```python
from build123d import *

# Parameters (mm, degrees)
SKETCH1_W                = 44.2976
SKETCH1_H                = 37.084
BOSS_EXTRUDE1_DEPTH      = 5.334
SKETCH2_W                = 6.1976
SKETCH2_H                = 5.334
CUT_EXTRUDE1_DEPTH       = 80.087198141
LPATTERN1_COUNT          = 3
LPATTERN1_PITCH          = 12.7
SKETCH3_W                = 5.334
SKETCH3_H                = 6.1976
CUT_EXTRUDE2_DEPTH       = 80.087198141
LPATTERN2_COUNT          = 2
LPATTERN2_PITCH          = 12.7
F_0_257_DIAMETER_HOLE1_D = 6.5278


with BuildPart() as part:
    # Sketch1 → Boss-Extrude1 (new body)
    with BuildSketch(Plane.XY):
        with Locations((50.0888, 13.208)):
            Rectangle(SKETCH1_W, SKETCH1_H)
    extrude(amount=-BOSS_EXTRUDE1_DEPTH)

    # Sketch2 → Cut-Extrude1 (cut, through all)
    with BuildSketch(Plane.XY):
        with Locations((62.7888, -2.667)):
            Rectangle(SKETCH2_W, SKETCH2_H)
    cut_extrude1 = extrude(amount=-CUT_EXTRUDE1_DEPTH, mode=Mode.SUBTRACT)

    # LPattern1: Cut-Extrude1 ×3
    with Locations(*[(-i * LPATTERN1_PITCH, 0, 0) for i in range(1, LPATTERN1_COUNT)]):
        add(cut_extrude1, mode=Mode.SUBTRACT)

    # Sketch3 → Cut-Extrude2 (cut, through all)
    with BuildSketch(Plane(origin=(0, 0, -5.334), x_dir=(-1, 0, 0), z_dir=(0, 0, -1))):
        with Locations((-69.5706, 9.6012)):
            Rectangle(SKETCH3_W, SKETCH3_H)
        with Locations((-30.607, 9.6012)):
            Rectangle(SKETCH3_W, SKETCH3_H)
    cut_extrude2 = extrude(amount=-CUT_EXTRUDE2_DEPTH, mode=Mode.SUBTRACT)

    # LPattern2: Cut-Extrude2 ×2
    with Locations(*[(0, i * LPATTERN2_PITCH, 0) for i in range(1, LPATTERN2_COUNT)]):
        add(cut_extrude2, mode=Mode.SUBTRACT)

    # F (0.257) Diameter Hole1 (through all)
    with Locations(Plane(origin=(0, 0, -5.334), x_dir=(-1, 0, 0), z_dir=(0, 0, -1))):
        with Locations((-59.6138, 15.875), (-40.5638, 15.875)):
            Hole(F_0_257_DIAMETER_HOLE1_D / 2)


solid = part.part
```
The model under review builds one solid part; all positions refer to its coordinate system, in mm. A direction names the side the tool comes from. Round coordinates to 2 decimals unless told otherwise and drop trailing zeros. Order: outer loops, then holes, each group sorted by start corner. A loop starts at its lowest first (then second) coordinate and runs counter-clockwise, first axis right, second up. Notation, with made-up numbers: (66.25, -14) -> (98.25, -14) arc R7 cw to (98.25, -9) -> close; hole circle Ø2 at (64.25, 8). An arc over 180 degrees is marked (long way). Use a Markdown table: item, result.
Q1. We need section D-D on y = 14.5. Write out the cut boundary in (x, z).
Values:
| item | result |
|---|---|
| outline | (27.94, -5.33) -> (37.6, -5.33) -> (37.6, 0) -> (27.94, 0) -> close; (43.52, -5.33) -> (56.65, -5.33) -> (56.65, 0) -> (43.52, 0) -> close; (62.57, -5.33) -> (72.24, -5.33) -> (72.24, 0) -> (62.57, 0) -> close |
Q2. Mouldability with a two-part tool opening along X and no side actions: class faces 4 (the flat face through (40.488, -3, -3)), 5 (the flat face through (69, -5.334, -3)), 6 (the flat face through (72.238, 16, -3)) as +X half, -X half, draft (parallel to the pull), parting line (faces both ways), or undercut.
Values:
| item | result |
|---|---|
| face 4 | undercut |
| face 5 | draft |
| face 6 | +X half |
Q3. For line 1 (Y direction, x = 67.5, z = -4.2); line 2 (X direction, y = 16.5, z = -2.6); line 3 (X direction, y = -1.5, z = -1.15), list the stretches that pass through material, from the lowest coordinate up.
Values:
| item | result |
|---|---|
| line 1 | y = -5.33 to 6.5, 12.7 to 19.2, 25.4 to 31.75 |
| line 2 | x = 27.94 to 37.36, 43.77 to 56.41, 62.82 to 72.24 |
| line 3 | x = 27.94 to 34.29, 40.49 to 46.99, 53.19 to 59.69, 65.89 to 72.24 |
Q4. Tool access review of faces 1 (the flat face through (31, 19.202, -3)), 2 (the flat face through (70, 12.7, -3)), 3 (the flat face through (63, 0, -3)): name each direction out of +Z, -Z, +X, -X, +Y, -Y from which nothing blocks a thin tool from reaching the whole face with its end or side.
Values:
| item | result |
|---|---|
| face 1 | +Z, -Z, -X |
| face 2 | +Z, -Z, +X |
| face 3 | +Z, -Z, -Y |
Q5. We need section C-C on z = -3.7. State how many separate pieces and enclosed holes the cut face has, then the cut area to 3 significant figures.
Values:
| item | result |
|---|---|
| separate pieces | 1 |
| enclosed holes | 2 |
| area | 1,340 mm^2 |
Q6. We need section B-B on x = 58.5. Write out the cut boundary in (y, z), then the cut area to 3 significant figures.
Values:
| item | result |
|---|---|
| outline | (-5.33, -5.33) -> (12.81, -5.33) -> (12.81, 0) -> (-5.33, 0) -> close; (18.94, -5.33) -> (31.75, -5.33) -> (31.75, 0) -> (18.94, 0) -> close |
| area | 165 mm^2 |
Q7. We need section A-A on y = -0.5. Write out the cut boundary in (x, z).
Values:
| item | result |
|---|---|
| outline | (27.94, -5.33) -> (34.29, -5.33) -> (34.29, 0) -> (27.94, 0) -> close; (40.49, -5.33) -> (46.99, -5.33) -> (46.99, 0) -> (40.49, 0) -> close; (53.19, -5.33) -> (59.69, -5.33) -> (59.69, 0) -> (53.19, 0) -> close; (65.89, -5.33) -> (72.24, -5.33) -> (72.24, 0) -> (65.89, 0) -> close |
Q8. Clearance check with flat-ended pins moving along their axes: P1, Ø2.5, axis at x = 36, z = -3, coming from the -Y side; P2, Ø2.5, axis at y = 10, z = -3, coming from the -X side. State where each tip first meets the part, or that it passes through.
Values:
| item | result |
|---|---|
| P1 | stops at y = 0 |
| P2 | stops at x = 33.27 |
